Part print with two shaded views. Sizes in mm from the minimum x, y, z corner. A direction names the side the tool comes from. Give positions to 0.01 mm unless a question says otherwise; leave off trailing zeros. Loops run counter-clockwise (first coordinate to the right, second up) from the corner with the lowest first, then second, coordinate; pieces in that order, holes last. Notation, with made-up numbers: M 72,31.5 L 106,31.5 A25 cw 106,43.5 Z; hole C 78.5,81.25 d8. An arc over 180 degrees is marked long. Answer as a JSON object with one key per item and string values. Group by question number.
1. Slice it at A-A (z = 1.15). List the corners of the cut face in (x, y), then the cut area to 3 significant figures.
2. Slice it at C-C (x = 6). List the corners of the cut face in (y, z), then the cut area to 3 significant figures.
3. Slice it at B-B (y = 3.4). List the corners of the cut face in (x, z).
4. Drill centre lines: line 1 along Y through (x, z) = (5, 2.8); line 2 along X through (y, z) = (0.2, 2.4); line 3 along Y through (x, z) = (1.75, 3.75). Where is each one in solid material? Low to high. Write a range as [from, to].
5. Drop flat-ended pins along their axis: pin 1 Ø0.8 at (y, z) = (4.5, 1.5) entering from -X; pin 2 Ø0.5 at (y, z) = (0.5, 2.5) entering from -X; pin 3 Ø1.5 at (x, z) = (1, 2) entering from +Y. Give the stop position or say it passes through.
6. 3-axis set-ups, long thin cutter, end or side, ignore diameter. For the marked faces 1, 2, 3 and 4: which of +Z, -Z, +X, -X, +Y, -Y reach the whole face in a straight line?
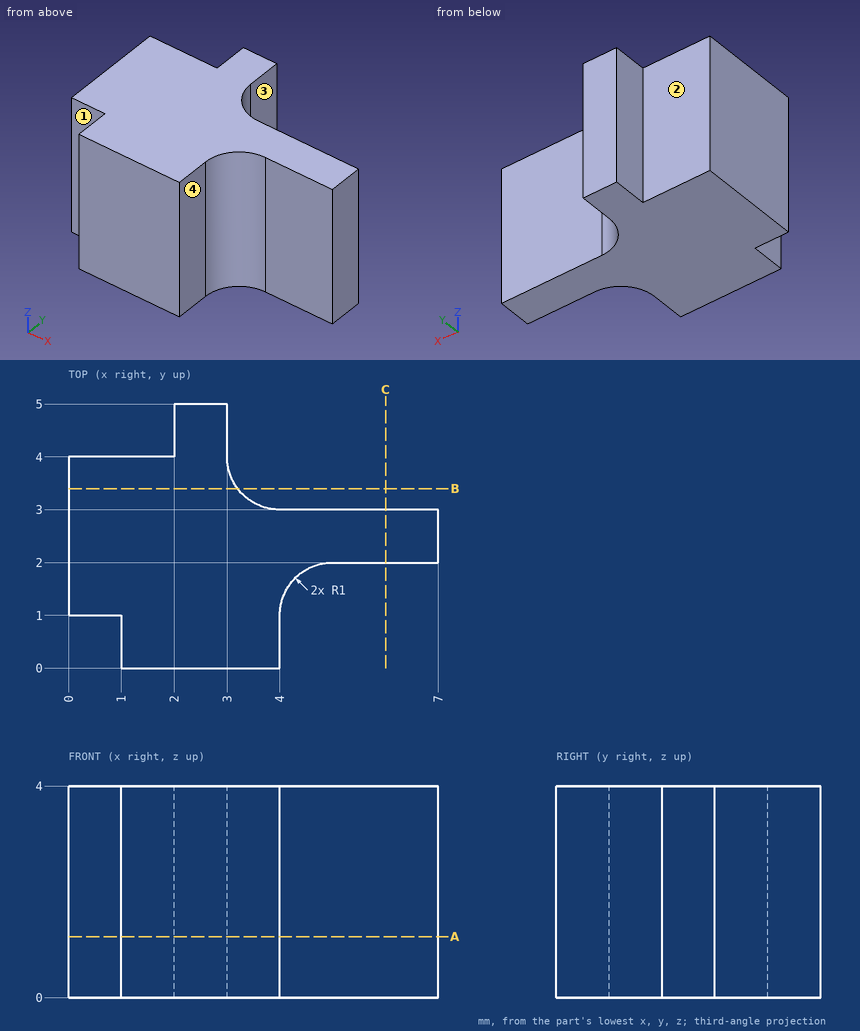
Established:
{
 "1": {"outline": "M 0,1 L 1,1 L 1,0 L 4,0 L 4,1 A1 cw 5,2 L 7,2 L 7,3 L 4,3 A1 cw 3,4 L 3,5 L 2,5 L 2,4 L 0,4 Z", "area": "18.4 mm^2"},
 "2": {"outline": "M 2,0 L 3,0 L 3,4 L 2,4 Z", "area": "4.00 mm^2"},
 "3": {"outline": "M 0,0 L 3.2,0 L 3.2,4 L 0,4 Z"},
 "4": {"line 1": "y = [2, 3]", "line 2": "x = [1, 4]", "line 3": "y = [0, 4]"},
 "5": {"pin 1": "stops at x = 2", "pin 2": "stops at x = 1", "pin 3": "stops at y = 4"},
 "6": {"face 1": "+Z, -Z, -X, -Y", "face 2": "+Z, -Z, -X, +Y", "face 3": "+Z, -Z, +X, +Y", "face 4": "+Z, -Z, +X, -Y"}
}
